The model under review builds one solid part; all positions refer to its coordinate system, in mm. Give positions to 0.01 mm unless a question says otherwise; leave off trailing zeros. Order: outer loops, then holes, each group sorted by start corner. A loop starts at its lowest first (then second) coordinate and runs counter-clockwise, first axis right, second up. Notation, with made-up numbers: (21.25, -34) - (70.25, -34) arc R10 cw to (70.25, -20) - close; hole circle Ø1 at (26, 68). An arc over 180 degrees is marked (long way). Use CSV: the item, a comma, the result in double quotes. Start each with the question number.
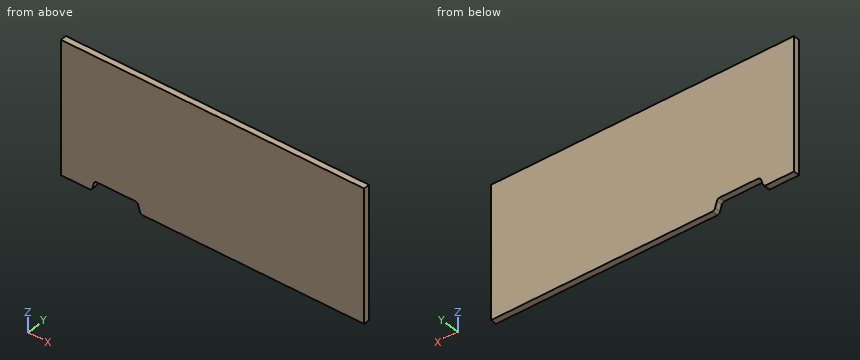
```python
from build123d import *

# Parameters (mm, degrees)
SKETCH1_W           = 628.65
SKETCH1_H           = 279.4
BOSS_EXTRUDE1_DEPTH = 12.7
CUT_EXTRUDE1_DEPTH  = 345.20573154
FILLET1_R           = 6.35


with BuildPart() as part:
    # Sketch1 → Boss-Extrude1 (new body)
    with BuildSketch(Plane(origin=(0, 0, 0), x_dir=(1, 0, 0), z_dir=(0, 1, 0))):
        Rectangle(SKETCH1_W, SKETCH1_H)
    extrude(amount=BOSS_EXTRUDE1_DEPTH)

    # Sketch2 → Cut-Extrude1 (cut, through all)
    with BuildSketch(Plane.XZ):
        Polygon((-149.225, -139.7), (-250.825, -139.7), (-244.475, -118.11), (-155.575, -118.11), align=None)
    extrude(amount=-CUT_EXTRUDE1_DEPTH, mode=Mode.SUBTRACT)

    # Fillet1
    fillet1_edges = [part.edges().sort_by_distance(p)[0] for p in [
        (-155.575, 6.35, -118.11),
        (-149.225, 6.35, -139.7),
        (-250.825, 6.35, -139.7),
        (-244.475, 6.35, -118.11),
    ]]
    fillet(fillet1_edges, radius=FILLET1_R)


solid = part.part
```
1. Consider section A-A (x = -183.5). Give the boundary of the cut face in (y, z).
2. Clearance check with a flat-ended pin moving along its axis: pin 1 (6 mm diameter, centred on x = -83, z = -20, fed in from -Y). State where the tip first meets the part, or that it passes through.
3. To check wall thickness, follow L1, parallel to X at y = 7.5, z = -123.5 (3 decimals); L2, parallel to Z at x = -219.5, y = 12; L3, parallel to Z at x = -155, y = 10. State the ranges of each line that lie inside material, in increasing order. Write a range as [from, to].
Answers follow:
1,outline,"(0, -118.11) - (12.7, -118.11) - (12.7, 139.7) - (0, 139.7) - close"
2,pin 1,"stops at y = 0"
3,L1,"x = [-314.325, -246.06], [-153.99, 314.325]"
3,L2,"z = [-118.11, 139.7]"
3,L3,"z = [-121, 139.7]"
